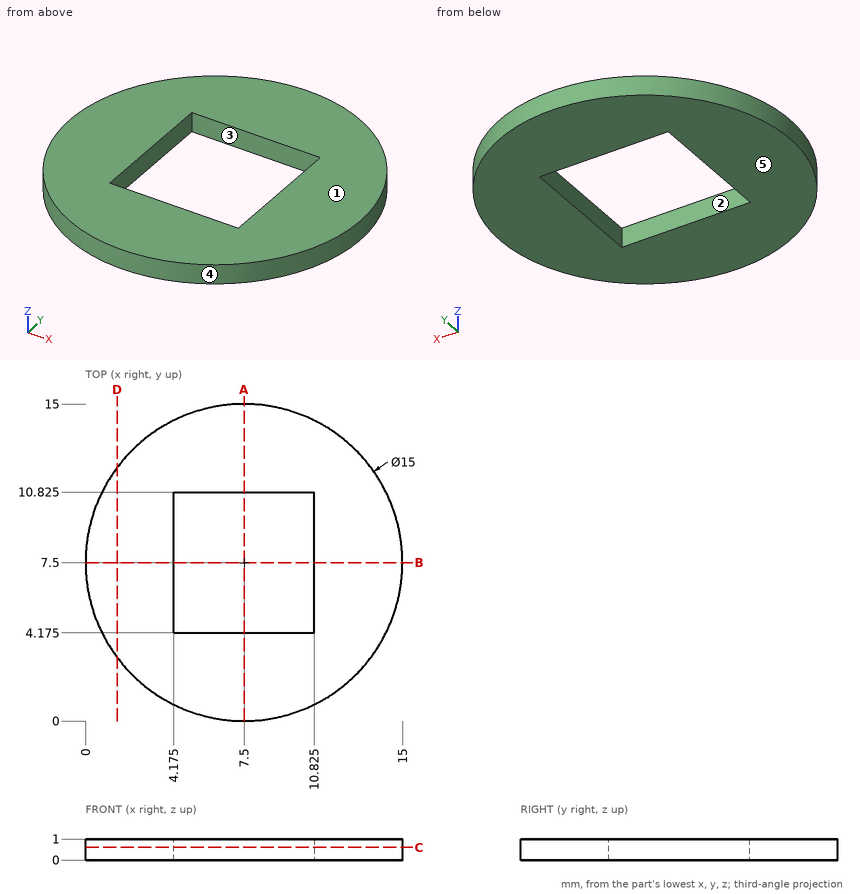
For this review, use the dimensioned drawing (mm, ordinates from the lowest corner) and the shaded views. A direction names the side the tool comes from. Coordinates: 2 decimals unless noted, no trailing zeros. Order: outer loops, then holes, each group sorted by start corner. A loop starts at its lowest first (then second) coordinate and runs counter-clockwise, first axis right, second up. Notation, with made-up numbers: (30, 39) - (44, 39) arc R17 cw to (44, 54) - close; hole circle Ø5 at (71.25, 37). An arc over 180 degrees is marked (long way). Use one line per item in the form item = value.
Q1. Consider section C-C (z = 0.6). Give the boundary of the cut face in (x, y) (3 decimals).
Checked values:
outline = circle Ø15 at (7.5, 7.5); hole (4.175, 4.175) - (10.825, 4.175) - (10.825, 10.825) - (4.175, 10.825) - close
Q2. For the marked faces 1 and 2, list the 3-axis set-ups (+Z, -Z, +X, -X, +Y, -Y) from which the entire face can be reached by the end or side of a thin tool; tool diameter is ignored.
Checked values:
face_1 = +Z, +X, -X, +Y, -Y
face_2 = +Z, -Z
Q3. Consider section D-D (x = 1.5). Give the boundary of the cut face in (y, z).
Checked values:
outline = (3, 0) - (12, 0) - (12, 1) - (3, 1) - close
Q4. For P1, Ø0.5, axis at x = 9, z = 0.5, coming from the +Y side; P2, Ø0.5, axis at y = 8, z = 0.5, coming from the +X side; P3, Ø0.5, axis at y = 6.5, z = 0.5, coming from the -X side, all flat-tipped, find the tip position at first contact; note any pin that passes through.
Checked values:
P1 = 14.9
P2 = 15
P3 = 0.04
Q5. Draft analysis for pull direction Y (two halves, no side actions). For the marked faces 3, 4 and 5, state which applies: +Y half, -Y half, draft (parallel to the pull), parting line (faces both ways), or undercut.
Checked values:
face_3 = undercut
face_4 = parting line
face_5 = draft
Q6. For probe 1 along Y at (x, z) = (7.75, 0.7) (3 decimals); probe 2 along X at (y, z) = (4.5, 0.5) (3 decimals); probe 3 along Y at (x, z) = (4.75, 0.9) (3 decimals), list the stretches that pass through material, from the lowest coordinate up. Write a range as from..to.
Checked values:
probe_1 = 0.004..4.175, 10.825..14.996
probe_2 = 0.626..4.175, 10.825..14.374
probe_3 = 0.522..4.175, 10.825..14.478
Q7. Consider section A-A (x = 7.5). Give the boundary of the cut face in (y, z) (3 decimals), then the cut area to 3 significant figures.
Checked values:
outline = (0, 0) - (4.175, 0) - (4.175, 1) - (0, 1) - close; (10.825, 0) - (15, 0) - (15, 1) - (10.825, 1) - close
area = 8.35 mm2
